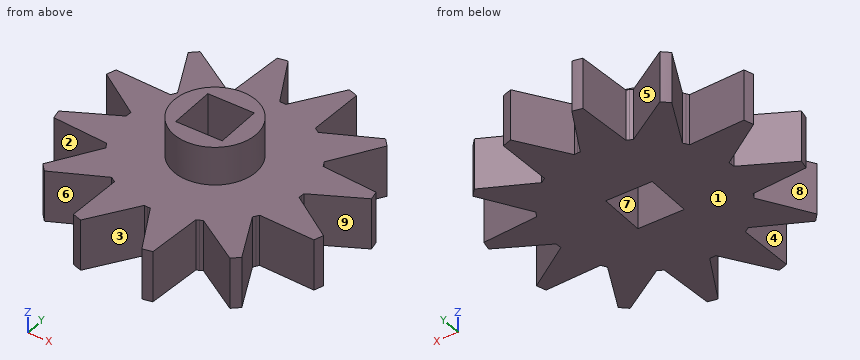
from build123d import *

# Parameters (mm, degrees)
F0_R            = 11
F1_DEPTH        = 4
F3_DEPTH        = 4.001
F3_COPIES_COUNT = 12
F5_R            = 3.2
F6_DEPTH        = 3
F7_W            = 3.6
F7_H            = 3.6
F8_DEPTH        = 7.001


# Not quite as in the source:
# - a pattern or mirror of a feature is missing from the dataset's text; its kind, count and spacing are read off the source's solid


with BuildPart() as f1:
    # F0 (on Top) → F1 (new body)
    with BuildSketch(Plane.XY):
        Circle(F0_R)
    extrude(amount=F1_DEPTH)

    # F2 (on face) → F3 (cut, through all)
    with BuildSketch(Plane.XY.offset(4)):
        with BuildLine():
            ThreePointArc((-3.3489182935, 6.1469298242), (-3.2411295194, 6.2044403002), (-3.1323534658, 6.2600608436))
            Line((-3.1323534658, 6.2600608436), (-4.922269732, 9.8372384685))
            ThreePointArc((-4.922269732, 9.8372384685), (-6.004235681, 9.2167865272), (-7.0090094429, 8.4778409179))
            Line((-7.0090094429, 8.4778409179), (-3.3489182935, 6.1469298242))
        make_face()
        with BuildLine():
            Line((-4.922269732, 9.8372384685), (-3.1323534658, 6.2600608436))
            ThreePointArc((-3.1323534658, 6.2600608436), (-3.022623267, 6.3137745118), (-2.9119723479, 6.3655649431))
            Line((-2.9119723479, 6.3655649431), (-2.5832151123, 10.6923804498))
            ThreePointArc((-2.5832151123, 10.6923804498), (-3.7770216625, 10.3312200326), (-4.922269732, 9.8372384685))
        make_face()
    f3 = extrude(amount=-F3_DEPTH, mode=Mode.SUBTRACT)

    # F3_copies: F3 ×12 about axis
    f3_copies_axis = Axis((0, 0, 0), (0, 0, 1))
    for i in range(1, F3_COPIES_COUNT):
        add(f3.rotate(f3_copies_axis, i * 360 / F3_COPIES_COUNT), mode=Mode.SUBTRACT)

    # F5 (on face) → F6 (join)
    with BuildSketch(Plane.XY.offset(4)):
        Circle(F5_R)
    extrude(amount=F6_DEPTH)

    # F7 (on face) → F8 (cut, through all)
    with BuildSketch(Plane.XY.offset(7)):
        Rectangle(F7_W, F7_H)
    extrude(amount=-F8_DEPTH, mode=Mode.SUBTRACT)


solid = f1.part
Verification items for the finished model (mm, model axes). Face numbers are marked on the shaded views. A direction names the side the tool comes from. Coordinates: 2 decimals unless noted, no trailing zeros. Order: outer loops, then holes, each group sorted by start corner. A loop starts at its lowest first (then second) coordinate and runs counter-clockwise, first axis right, second up.
1. Release check for a two-part mould opening along Y. For the marked faces 1, 2, 3 and 4 record: +Y half, -Y half, draft (parallel to the pull), parting line (faces both ways), or undercut.
Results found:
face 1: draft
face 2: undercut
face 3: -Y half
face 4: undercut
2. Go/stop test with flat-tipped pins: pin 1 Ø5 at (x, y) = (1.5, 7.5) entering from -Z; pin 2 Ø4 at (x, z) = (0.5, 4) entering from +Y; pin 3 Ø1.1 at (y, z) = (-0.5, 3) entering from -X; pin 4 Ø4 at (x, z) = (-0.5, 4) entering from -Y. Record where each tip stops, or that it passes through.
Results found:
pin 1: stops at z = 0
pin 2: stops at y = 10.21
pin 3: stops at x = -9.35
pin 4: stops at y = -10.21
3. Set-up check for the marked faces 5, 6, 7, 8 and 9: record each of +Z, -Z, +X, -X, +Y, -Y from which the full face is reachable in a straight line by a thin tool's end or side.
Results found:
face 5: +Z, -Z, +Y
face 6: +Z, -Z, -Y
face 7: +Z, -Z
face 8: +Z, -Z, -X
face 9: +Z, -Z, +X
4. Sectioned sample at A-A, the plane z = 6.5. Record the cut outline in (x, y), and give its area (3 significant figures).
Results found:
outline: circle Ø6.4 at (0, 0); hole (-1.8, -1.8) - (1.8, -1.8) - (1.8, 1.8) - (-1.8, 1.8) - close
area: 19.2 mm2
5. Scan lines: line 1 (X direction, y = -7.75, z = 1.5); line 2 (X direction, y = -9, z = 1.5); line 3 (Z direction, x = 0.75, y = 5.5). Record each from-to range of solid material in increasing order.
Results found:
line 1: x = -3.73 to -1.19, 0.22 to 2.81, 5.87 to 7.48
line 2: x = -3.78 to -2.05, 0.87 to 2.71
line 3: z = 0 to 4
6. Sectioned sample at B-B, the plane x = 4.5. Record the cut outline in (y, z), and give its area (3 significant figures).
Results found:
outline: (-6.88, 0) - (5.92, 0) - (5.92, 4) - (-6.88, 4) - close
area: 51.2 mm2
